Could you check a few things on this model? Use its own coordinates, in mm. A direction names the side the tool comes from. Give positions to 0.01 mm unless a question says otherwise; leave off trailing zeros. Write each loop counter-clockwise with the first axis right and the second up, starting at its lowest first coordinate (ties: lowest second). Pieces come first, ordered by that corner, then holes. Notation, with made-up numbers: (-32.5, -4) - (-16.5, -4) arc R30 cw to (-16.5, 31) - close; hole circle Ø1 at (-38, -10.75). An arc over 180 degrees is marked (long way). Write item = value, one per line.
from build123d import *

# Parameters (mm, degrees)
SKETCH1_W           = 244
SKETCH1_H           = 158.15
BOSS_EXTRUDE1_DEPTH = 5
CUT_EXTRUDE1_DEPTH  = 10
CUT_EXTRUDE2_DEPTH  = 10
SKETCH4_R           = 2.5
CUT_EXTRUDE3_DEPTH  = 10


with BuildPart() as part:
    # Sketch1 → Boss-Extrude1 (new body)
    with BuildSketch(Plane.XY):
        with Locations((14.8, -10.925)):
            Rectangle(SKETCH1_W, SKETCH1_H)
    extrude(amount=BOSS_EXTRUDE1_DEPTH)

    # Sketch2 → Cut-Extrude1 (cut)
    with BuildSketch(Plane(origin=(0, 0, 0), x_dir=(-1, 0, 0), z_dir=(0, 0, -1))):
        Polygon((-136.8, 45.15), (-129.8, 45.15), (-129.8, 45.9), (-127.4, 45.9), (-127.4, 45.15), (-119.8, 45.15), (-119.8, 41.15), (-127.4, 41.15), (-127.4, 40.4), (-129.8, 40.4), (-129.8, 41.15), (-136.8, 41.15), align=None)
        Polygon((-129.8, -63), (-136.8, -63), (-136.8, -67), (-129.8, -67), (-129.8, -67.75), (-127.4, -67.75), (-127.4, -67), (-119.8, -67), (-119.8, -63), (-127.4, -63), (-127.4, -62.25), (-129.8, -62.25), align=None)
        Polygon((100.2, 41.15), (107.2, 41.15), (107.2, 45.15), (100.2, 45.15), (100.2, 45.9), (97.8, 45.9), (97.8, 45.15), (90.2, 45.15), (90.2, 41.15), (97.8, 41.15), (97.8, 40.4), (100.2, 40.4), align=None)
        Polygon((107.2, -67), (100.2, -67), (100.2, -67.75), (97.8, -67.75), (97.8, -67), (90.2, -67), (90.2, -63), (97.8, -63), (97.8, -62.25), (100.2, -62.25), (100.2, -63), (107.2, -63), align=None)
    extrude(amount=-CUT_EXTRUDE1_DEPTH, mode=Mode.SUBTRACT)

    # Sketch3 → Cut-Extrude2 (cut)
    with BuildSketch(Plane(origin=(0, 0, 0), x_dir=(-1, 0, 0), z_dir=(0, 0, -1))):
        with BuildLine():
            Line((-106.8, 38.15), (-46.8, 38.15))
            ThreePointArc((-46.8, 38.15), (-41.8, 33.15), (-46.8, 28.15))
            Line((-46.8, 28.15), (-106.8, 28.15))
            ThreePointArc((-106.8, 28.15), (-111.8, 33.15), (-106.8, 38.15))
        make_face()
        with BuildLine():
            Line((-46.8, -50), (-106.8, -50))
            ThreePointArc((-106.8, -50), (-111.8, -55), (-106.8, -60))
            Line((-106.8, -60), (-46.8, -60))
            ThreePointArc((-46.8, -60), (-41.8, -55), (-46.8, -50))
        make_face()
        with BuildLine():
            Line((77.2, -60), (17.2, -60))
            ThreePointArc((17.2, -60), (12.2, -55), (17.2, -50))
            Line((17.2, -50), (77.2, -50))
            ThreePointArc((77.2, -50), (82.2, -55), (77.2, -60))
        make_face()
        with BuildLine():
            Line((17.2, 28.15), (77.2, 28.15))
            ThreePointArc((77.2, 28.15), (82.2, 33.15), (77.2, 38.15))
            Line((77.2, 38.15), (17.2, 38.15))
            ThreePointArc((17.2, 38.15), (12.2, 33.15), (17.2, 28.15))
        make_face()
    extrude(amount=-CUT_EXTRUDE2_DEPTH, mode=Mode.SUBTRACT)

    # Sketch4 → Cut-Extrude3 (cut)
    with BuildSketch(Plane(origin=(0, 0, 0), x_dir=(-1, 0, 0), z_dir=(0, 0, -1))):
        with Locations((50.2, 48.15)):
            Circle(SKETCH4_R)
        with Locations((-79.8, 48.15)):
            Circle(SKETCH4_R)
        with Locations((-124.8, -75.004567899)):
            Circle(SKETCH4_R)
        with Locations((95.2, -75.004567899)):
            Circle(SKETCH4_R)
    extrude(amount=-CUT_EXTRUDE3_DEPTH, mode=Mode.SUBTRACT)


solid = part.part
1. If we section it at C-C, the plane y = -55: Please give me the cut outline in (x, z), and give its area (3 significant figures).
Filled sheet:
outline = (-107.2, 0) - (-82.2, 0) - (-82.2, 5) - (-107.2, 5) - close; (-12.2, 0) - (41.8, 0) - (41.8, 5) - (-12.2, 5) - close; (111.8, 0) - (136.8, 0) - (136.8, 5) - (111.8, 5) - close
area = 520 mm2
2. If we section it at D-D, the plane x = -50.2: Please give me the cut outline in (y, z).
Filled sheet:
outline = (-90, 0) - (-60, 0) - (-60, 5) - (-90, 5) - close; (-50, 0) - (28.15, 0) - (28.15, 5) - (-50, 5) - close; (38.15, 0) - (45.65, 0) - (45.65, 5) - (38.15, 5) - close; (50.65, 0) - (68.15, 0) - (68.15, 5) - (50.65, 5) - close
3. Thinking about a two-plate mould opening in Y: for faces 1 (the face through (136.8, -12, 2)), 2 (the face through (-94, 41.15, 2)), which applies, pulls with the +Y half, pulls with the -Y half, needs draft (parallel to the pull), parting line crosses it, or undercut?
Filled sheet:
face_1 = needs draft
face_2 = undercut
4. If we section it at A-A, the plane x = 96: Please give me the cut outline in (y, z).
Filled sheet:
outline = (-90, 0) - (-60, 0) - (-60, 5) - (-90, 5) - close; (-50, 0) - (28.15, 0) - (28.15, 5) - (-50, 5) - close; (38.15, 0) - (68.15, 0) - (68.15, 5) - (38.15, 5) - close
5. If we section it at B-B, the plane x = -95.2: Please give me the cut outline in (y, z).
Filled sheet:
outline = (-90, 0) - (-77.5, 0) - (-77.5, 5) - (-90, 5) - close; (-72.5, 0) - (-67, 0) - (-67, 5) - (-72.5, 5) - close; (-63, 0) - (41.15, 0) - (41.15, 5) - (-63, 5) - close; (45.15, 0) - (68.15, 0) - (68.15, 5) - (45.15, 5) - close
6. I need wall thicknesses on line 1 (Y direction, x = 124.8, z = 2.6); line 2 (Y direction, x = -33.5, z = 1.75); line 3 (Y direction, x = 79.8, z = 3.5). Which ranges of each line are inside material? Lowest first, please.
Filled sheet:
line_1 = -90 to -77.5, -72.5 to -67, -63 to 41.15, 45.15 to 68.15
line_2 = -90 to -60, -50 to 28.15, 38.15 to 68.15
line_3 = -90 to -60, -50 to 28.15, 38.15 to 45.65, 50.65 to 68.15
7. Which directions (+Z, -Z, +X, -X, +Y, -Y) give clear straight access to the entire face, cutting with the end or side of a thin tool? Please do faces 3 (the face through (41.8, -55.1, 2.5)), 4 (the face through (133, -63, 2)), 5 (the face through (-104, -67, 2)).
Filled sheet:
face_3 = +Z, -Z
face_4 = +Z, -Z, +X
face_5 = +Z, -Z, -X
